```python
from build123d import *

# Parameters (mm, degrees)
MODEL_W             = 4.499998054
MODEL_H             = 21.693928328
MODEL_H_2           = 21.693787217
BOSS_EXTRUDE1_DEPTH = 4.5


with BuildPart() as part:
    # Model → Boss-Extrude1 (new body)
    with BuildSketch(Plane.XY):
        Polygon((760.050761477, -825.00268896), (747.275655091, -825.00268896), (747.275655091, -829.502687015), (722.525753986, -829.502687015), (718.025755932, -829.502687015), (718.025755932, -846.202798955), (722.525753986, -846.202798955), (722.525753986, -867.402520894), (718.025755932, -867.402520894), (718.025755932, -876.311006448), (738.62589676, -876.311006448), (738.62589676, -875.061150059), (741.125997592, -875.061150059), (741.125997592, -876.311006448), (743.625922036, -876.311006448), (743.625922036, -879.410935336), (741.125997592, -879.410935336), (741.125997592, -880.660791724), (738.62589676, -880.660791724), (738.62589676, -879.410935336), (718.025755932, -879.410935336), (718.025755932, -888.602772), (722.525753986, -888.602772), (722.525753986, -909.802529217), (718.025755932, -909.802529217), (718.025755932, -926.502288379), (747.275655091, -926.502288379), (747.275655091, -931.002251156), (760.050761477, -931.002251156), (760.050761477, -927.30221199), (763.750800642, -927.30221199), (763.750800642, -931.002251156), (776.52555425, -931.002251156), (776.52555425, -926.502288379), (797.525462856, -926.502288379), (797.525462856, -931.002251156), (818.525759518, -931.002251156), (818.525759518, -926.502288379), (839.525668123, -926.502288379), (839.525668123, -931.002251156), (860.525612007, -931.002251156), (860.525612007, -926.502288379), (881.525873391, -926.502288379), (881.525873391, -931.002251156), (902.525781997, -931.002251156), (902.525781997, -926.502288379), (923.52572588, -926.502288379), (923.52572588, -931.002251156), (944.525634486, -931.002251156), (944.525634486, -926.502288379), (965.52557837, -926.502288379), (965.52557837, -931.002251156), (978.300649478, -931.002251156), (978.300649478, -927.30221199), (982.000688643, -927.30221199), (982.000688643, -931.002251156), (994.775795029, -931.002251156), (994.775795029, -926.502288379), (1024.025694188, -926.502288379), (1024.025694188, -909.802529217), (1019.525696134, -909.802529217), (1019.525696134, -888.602772), (1024.025694188, -888.602772), (1024.025694188, -879.852225058), (1020.325655023, -879.852225058), (1020.325655023, -876.152715059), (1024.025694188, -876.152715059), (1024.025694188, -867.402520894), (1019.525696134, -867.402520894), (1019.525696134, -846.202798955), (1024.025694188, -846.202798955), (1024.025694188, -829.502687015), (1019.525696134, -829.502687015), (994.775442251, -829.502687015), (994.775442251, -825.00268896), (982.000688643, -825.00268896), (982.000688643, -828.702728126), (978.300649478, -828.702728126), (978.300649478, -825.00268896), (965.52557837, -825.00268896), (965.52557837, -829.502687015), (944.525634486, -829.502687015), (944.525634486, -825.00268896), (923.52572588, -825.00268896), (923.52572588, -829.502687015), (902.525429219, -829.502687015), (902.525429219, -825.00268896), (881.525520613, -825.00268896), (881.525520613, -829.502687015), (860.525612007, -829.502687015), (860.525612007, -825.00268896), (839.525668123, -825.00268896), (839.525668123, -829.502687015), (818.525759518, -829.502687015), (818.525759518, -825.00268896), (797.525462856, -825.00268896), (797.525462856, -829.502687015), (776.52555425, -829.502687015), (776.52555425, -825.00268896), (763.750800642, -825.00268896), (763.750800642, -828.702728126), (760.050761477, -828.702728126), align=None)
        with Locations((921.275726853, -856.555380341)):
            Rectangle(MODEL_W, MODEL_H, mode=Mode.SUBTRACT)
        with Locations((921.275726853, -898.955635608)):
            Rectangle(MODEL_W, MODEL_H_2, mode=Mode.SUBTRACT)
        with BuildLine():
            add(Edge.make_bspline(
                [(752.476022867, -917.002758937), (751.564797868, -917.002758937), (750.826187035, -916.264148104), (750.826187035, -915.352570327), (750.826187035, -914.441698105), (751.564797868, -913.702381716), (752.476022867, -913.702381716)],
                knots=[2, 2, 2, 2, 3, 3, 3, 4, 4, 4, 4], degree=3))
            add(Edge.make_bspline(
                [(752.476022867, -913.702381716), (753.387247867, -913.702381716), (754.126246756, -914.441698105), (754.126246756, -915.352570327), (754.126246756, -916.264148104), (753.387247867, -917.002758937), (752.476022867, -917.002758937)],
                knots=[0, 0, 0, 0, 1, 1, 1, 2, 2, 2, 2], degree=3))
        make_face(mode=Mode.SUBTRACT)
        with BuildLine():
            add(Edge.make_bspline(
                [(752.476022867, -846.739021177), (751.564797868, -846.739021177), (750.826187035, -846.000375066), (750.826187035, -845.088797289), (750.826187035, -844.177925067), (751.564797868, -843.438608678), (752.476022867, -843.438608678)],
                knots=[2, 2, 2, 2, 3, 3, 3, 4, 4, 4, 4], degree=3))
            add(Edge.make_bspline(
                [(752.476022867, -843.438608678), (753.387247867, -843.438608678), (754.126246756, -844.177925067), (754.126246756, -845.088797289), (754.126246756, -846.000375066), (753.387247867, -846.739021177), (752.476022867, -846.739021177)],
                knots=[0, 0, 0, 0, 1, 1, 1, 2, 2, 2, 2], degree=3))
        make_face(mode=Mode.SUBTRACT)
        with BuildLine():
            add(Edge.make_bspline(
                [(854.523909509, -917.002758937), (853.61282562, -917.002758937), (852.874214787, -916.264148104), (852.874214787, -915.352570327), (852.874214787, -914.441698105), (853.61282562, -913.702381716), (854.523909509, -913.702381716)],
                knots=[2, 2, 2, 2, 3, 3, 3, 4, 4, 4, 4], degree=3))
            add(Edge.make_bspline(
                [(854.523909509, -913.702381716), (855.435452008, -913.702381716), (856.174274508, -914.441698105), (856.174274508, -915.352570327), (856.174274508, -916.264148104), (855.435452008, -917.002758937), (854.523909509, -917.002758937)],
                knots=[0, 0, 0, 0, 1, 1, 1, 2, 2, 2, 2], degree=3))
        make_face(mode=Mode.SUBTRACT)
        with BuildLine():
            add(Edge.make_bspline(
                [(854.523909509, -846.738844788), (853.61282562, -846.738844788), (852.874214787, -846.000198677), (852.874214787, -845.088656178), (852.874214787, -844.177748678), (853.61282562, -843.438432289), (854.523909509, -843.438432289)],
                knots=[2, 2, 2, 2, 3, 3, 3, 4, 4, 4, 4], degree=3))
            add(Edge.make_bspline(
                [(854.523909509, -843.438432289), (855.435452008, -843.438432289), (856.174274508, -844.177748678), (856.174274508, -845.088656178), (856.174274508, -846.000198677), (855.435452008, -846.738844788), (854.523909509, -846.738844788)],
                knots=[0, 0, 0, 0, 1, 1, 1, 2, 2, 2, 2], degree=3))
        make_face(mode=Mode.SUBTRACT)
    extrude(amount=BOSS_EXTRUDE1_DEPTH)


solid = part.part
```
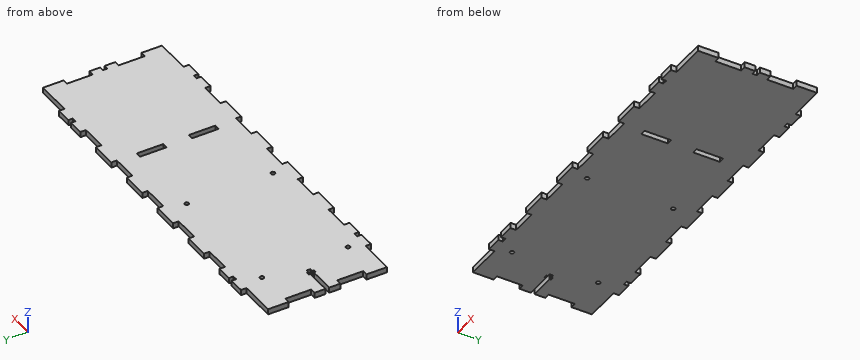
Could you check a few things on this model? Use its own coordinates, in mm. Round coordinates to 2 decimals unless told otherwise and drop trailing zeros. Order: outer loops, then holes, each group sorted by start corner. A loop starts at its lowest first (then second) coordinate and runs counter-clockwise, first axis right, second up. Notation, with made-up numbers: M 22.5,-18 L 79.5,-18 A20 cw 79.5,-11 Z; hole C 18,49.5 d1. An arc over 180 degrees is marked long. One line per question, with ' | ' between items. Start each with the question number.
(1) Suppose I cut it at C-C on z = 2.85. Count the separate pieces of the cut face and the enclosed holes in it, then the cut area to 3 significant figures.
(2) For P1, Ø1.3, axis at y = -827.5, z = 1.5, coming from the +X side; P2, Ø1.2, axis at x = 742, z = 1.5, coming from the -Y side; P3, Ø2, axis at x = 720, z = 2, coming from the +Y side, each with a flat end and sliding along its axis, tell me the tip position at first contact or that it passes through.
(3) Please list where these lines run through material, in increasing order: line 1 along X through (y, z) = (-900, 4.35); line 2 along Y through (x, z) = (980.5, 3.7); line 3 along X through (y, z) = (-877, 3.6).
(4) Suppose I cut it at B-B on x = 999.5. List the corners of the cut face in (y, z) for me, then the cut area to 3 significant figures.
(5) Suppose I cut it at A-A on y = -864. List the corners of the cut face in (x, z) for me.
Geometry results:
1) separate pieces: 1 | enclosed holes: 6 | area: 30,200 mm²
2) P1: x = 994.78 | P2: y = -926.5 | P3: y = -829.5
3) line 1: 722.53 to 919.03, 923.53 to 1019.53 | line 2: -927.3 to -828.7 | line 3: 743.63 to 1020.33
4) outline: M -926.5,0 L -829.5,0 L -829.5,4.5 L -926.5,4.5 Z | area: 436 mm²
5) outline: M 722.53,0 L 919.03,0 L 919.03,4.5 L 722.53,4.5 Z; M 923.53,0 L 1019.53,0 L 1019.53,4.5 L 923.53,4.5 Z
